Drawing for the job (mm, zero at the part's lowest x, y, z). Round coordinates to 2 decimals unless told otherwise and drop trailing zeros. Write each loop counter-clockwise with the first axis right and the second up, starting at its lowest first coordinate (ties: lowest second). Pieces come first, ordered by that corner, then holes.
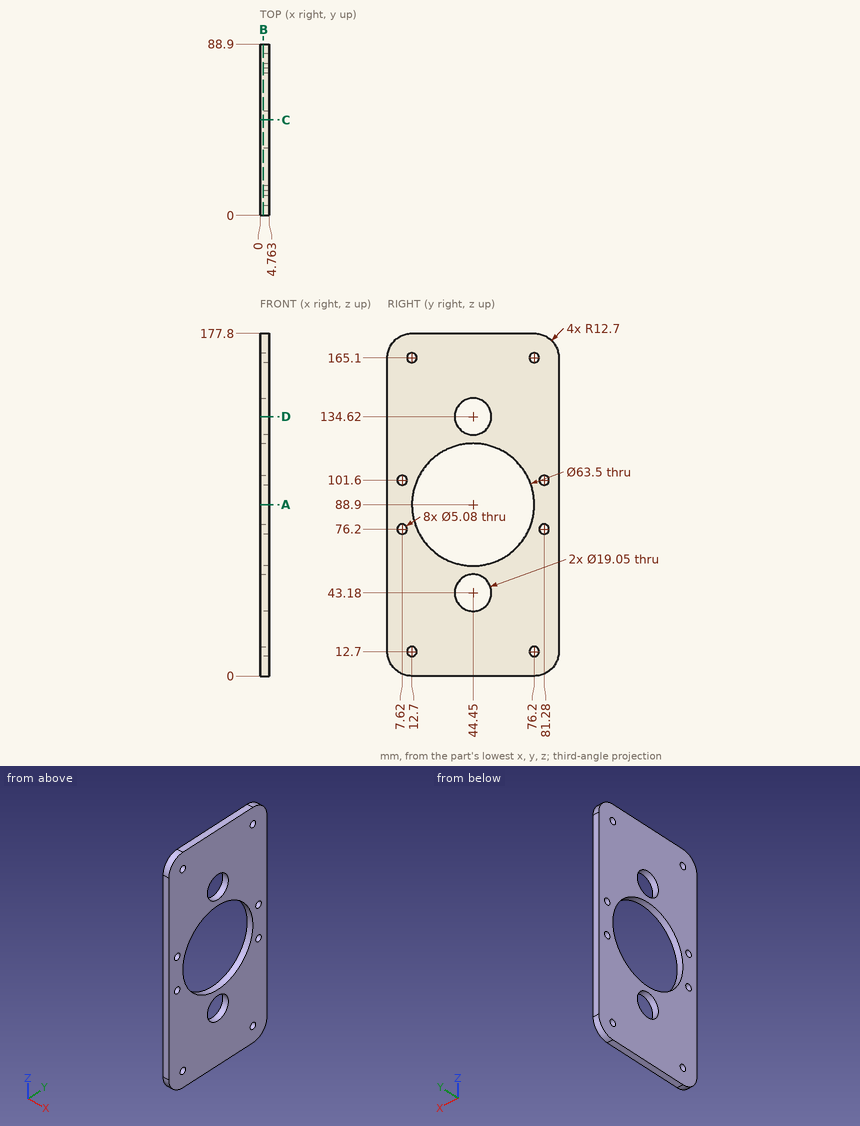
Q1. Wall check: line 1 (Y direction, x = 1.75, z = 101.6); line 2 (Z direction, x = 1.45, y = 81.28); line 3 (Z direction, x = 1.1, y = 46). Give the ranges that are in metal, low to high.
Q2. Saw through at B-B, the plane x = 1.6. Give the number of separate pieces and of enclosed holes in the cut face, and give its area (3 significant figures).
Q3. Saw through at C-C, the plane y = 49.5. Write the cut outline in (x, z) (1 decimal).
Q4. Saw through at A-A, the plane z = 88.9. Write the cut outline in (x, y), and give its area (3 significant figures).
Q5. Saw through at D-D, the plane z = 134.62. Write the cut outline in (x, y) (1 decimal).
Computed:
1. line 1: y = 0 to 5.08, 10.16 to 15.35, 73.55 to 78.74, 83.82 to 88.9
1. line 2: z = 1.06 to 73.66, 78.74 to 99.06, 104.14 to 176.74
1. line 3: z = 0 to 33.78, 52.58 to 57.19, 120.61 to 125.22, 144.02 to 177.8
2. separate pieces: 1
2. enclosed holes: 11
2. area: 11,800 mm2
3. outline: (0, 0) - (4.8, 0) - (4.8, 35.1) - (0, 35.1) - close; (0, 51.3) - (4.8, 51.3) - (4.8, 57.6) - (0, 57.6) - close; (0, 120.2) - (4.8, 120.2) - (4.8, 126.5) - (0, 126.5) - close; (0, 142.7) - (4.8, 142.7) - (4.8, 177.8) - (0, 177.8) - close
4. outline: (0, 0) - (4.76, 0) - (4.76, 12.7) - (0, 12.7) - close; (0, 76.2) - (4.76, 76.2) - (4.76, 88.9) - (0, 88.9) - close
4. area: 121 mm2
5. outline: (0, 0) - (4.8, 0) - (4.8, 34.9) - (0, 34.9) - close; (0, 54) - (4.8, 54) - (4.8, 88.9) - (0, 88.9) - close
